Source: CAD feature listing. Evaluate the final solid. Frame: model axes, mm. A direction names the side the tool comes from. Give positions to 0.01 mm unless a question says otherwise; leave off trailing zeros. Loops run counter-clockwise (first coordinate to the right, second up) from the corner with the lowest first, then second, coordinate; pieces in that order, holes last. Notation, with made-up numbers: (11, -40) - (55, -40) arc R30 cw to (55, -11) - close; hole circle Ø1 at (-23, 22.25). An arc over 180 degrees is marked (long way). Put each result on its own line as item: value.
Autodesk Inventor part; units mm, degrees
ref_plane "Work Plane1" through (0, 304.8, 0) normal (0, -1, 0) x (1, 0, 0)
ref_plane "YZ Plane" through (0, 0, 0) normal (1, 0, 0) x (0, 1, 0)
ref_plane "XZ Plane" through (0, 0, 0) normal (0, 1, 0) x (-1, 0, 0)
sketch "Sketch1" plane through (0, 0, 0) normal (0, 0, 1) x (1, 0, 0)
  line L0 (0, 0) -> (914.4, 0)
  line L1 (914.4, 0) -> (914.4, 609.6)
  line L2 (914.4, 609.6) -> (0, 609.6)
  line L3 (0, 609.6) -> (0, 0)
  line L4 (12.7, 12.7) -> (901.7, 12.7)
  line L5 (901.7, 12.7) -> (901.7, 596.9)
  line L6 (901.7, 596.9) -> (12.7, 596.9)
  line L7 (12.7, 596.9) -> (12.7, 12.7)
  dimension "d0" = 609.6
  dimension "d1" = 914.4
  dimension "d2" = 12.7
  dimension "d3" = 12.7
  dimension "d4" = 12.7
  dimension "d5" = 12.7
extrude "Extrusion1" add sketch "Sketch1" along normal blind 406.4
extrude "Extrusion2" add sketch "Sketch1" along normal blind 12.7 contours L7 L6 L5 L4
ref_plane "Work Plane1" through (0, 304.8, 0) normal (0, -1, 0) x (1, 0, 0)
equation "\"d0\" = length"
equation "\"d1\" = width"
equation "\"d2\" = thickness"
equation "\"d3\" = thickness"
equation "\"d4\" = thickness"
equation "\"d5\" = thickness"
equation "\"d6\" = height"
equation "\"d8\" = thickness"
equation "\"length\" = 609.6"
equation "\"width\" = 914.4"
equation "\"height\" = 406.4"
equation "\"thickness\" = 12.7"
properties part number "box"
1) Access query for faces 1 (the flat face through (0, 309, 200)), 2 (the flat face through (901.7, 301, 207)). Directions: +Z, -Z, +X, -X, +Y, -Y. A direction counts if a zero-diameter tool reaches every point of the face in a straight line with its end or side. Return the directions, or none.
Check result:
face 1: +Z, -Z, -X, +Y, -Y
face 2: +Z
2) Section query B-B, the plane x = 465.5. Output: boundary loops of the cut face in (y, z), plus the area to 3 significant figures.
Check result:
outline: (0, 0) - (609.6, 0) - (609.6, 406.4) - (596.9, 406.4) - (596.9, 12.7) - (12.7, 12.7) - (12.7, 406.4) - (0, 406.4) - close
area: 17,700 mm²
3) Section query C-C, the plane y = 155.5. Output: boundary loops of the cut face in (x, z).
Check result:
outline: (0, 0) - (914.4, 0) - (914.4, 406.4) - (901.7, 406.4) - (901.7, 12.7) - (12.7, 12.7) - (12.7, 406.4) - (0, 406.4) - close
4) Section query A-A, the plane z = 37. Output: boundary loops of the cut face in (x, y).
Check result:
outline: (0, 0) - (914.4, 0) - (914.4, 609.6) - (0, 609.6) - close; hole (12.7, 12.7) - (901.7, 12.7) - (901.7, 596.9) - (12.7, 596.9) - close
5) Pin query (flat end, axial travel): P1, Ø3, axis at x = 682, y = 429, coming from the +Z side. Return the tip coordinate at first contact, or that it passes through.
Check result:
P1: z = 12.7
6) Mould query, pull axis Y, two halves, no side actions, for faces 3 (the flat face through (464, 609.6, 200)), 4 (the flat face through (455, 600, 406.4)), 5 (the flat face through (451, 12.7, 207)). Classes: pulls with the +Y half, pulls with the -Y half, needs draft (parallel to the pull), parting line crosses it, or undercut.
Check result:
face 3: pulls with the +Y half
face 4: needs draft
face 5: undercut
7) Material intervals for line 1 along Y through (x, z) = (836, 99.5); line 2 along X through (y, z) = (214.5, 274.5); line 3 along Z through (x, y) = (359.5, 164), sorted ascending. Write a range as [from, to].
Check result:
line 1: [0, 12.7], [596.9, 609.6]
line 2: [0, 12.7], [901.7, 914.4]
line 3: [0, 12.7]
